Design review of the part built by this model. Coordinates are the model's own, in mm. A direction names the side the tool comes from. Give positions to 0.01 mm unless a question says otherwise; leave off trailing zeros. Order: outer loops, then holes, each group sorted by start corner. A loop starts at its lowest first (then second) coordinate and runs counter-clockwise, first axis right, second up. Notation, with made-up numbers: (-2, -35.75) -> (43, -35.75) arc R27 ccw to (43, 3.25) -> close; hole circle Ø4 at (71.5, -10). An arc over 180 degrees is marked (long way). One line per item, written item: value. Start each with the question number.
1) Consider section D-D (x = 3.5). State the section outline as (y, z) points, plus the area to 3 significant figures.
2) Consider section A-A (y = 0.9). State the section outline as (x, z) points, plus the area to 3 significant figures.
3) Consider section B-B (x = -15.25). State the section outline as (y, z) points, plus the area to 3 significant figures.
4) For pin 1 (11 mm diameter, centred on x = 3.5, z = -4, fed in from +Y); pin 2 (1 mm diameter, centred on y = 3, z = 3, fed in from -X); pin 3 (0.5 mm diameter, centred on x = 6.5, y = 2.5, fed in from +Z); pin 4 (1.1 mm diameter, centred on y = 2.5, z = 15.5, fed in from -X), all flat-tipped, find the tip position at first contact; note any pin that passes through.
5) The part is to be moulded in two halves that separate along Z. For faces 1 (the face through (0, 0, 0)), 2 (the face through (15.32, 0.86, -16.75)), 3 (the face through (-15.18, 0.86, -16.75)), 4 (the face through (17.43, 0.86, 17.4)), say which applies: released by +Z, released by -Z, zero draft, split by the parting line, or undercut.
6) Consider section C-C (z = -5.5). State the section outline as (x, y) points, plus the area to 3 significant figures.
7) Tool access review of faces 5 (the face through (7, 3, 15)), 6 (the face through (0, 1, -18)): name each direction out of +Z, -Z, +X, -X, +Y, -Y from which nothing blocks a thin tool from reaching the whole face with its end or side.
8) Wall thickness on line 1 along X through (y, z) = (1.45, 15.25); line 2 along Y through (x, z) = (0.5, -12): over which ranges is each line inside the solid? List them lowest first. Write a range as from..to.
from build123d import *

# Parameters (mm, degrees)
SKETCH2_R           = 1.5
BOSS_EXTRUDE1_DEPTH = 1.75
BOSS_EXTRUDE2_DEPTH = 3
BOSS_EXTRUDE3_DEPTH = 0.5
SKETCH6_R           = 0.25
CUT_EXTRUDE1_DEPTH  = 38.316216314


with BuildPart() as part:
    # Sketch2 → Boss-Extrude1 (new body)
    with BuildSketch(Plane(origin=(0, 0, 0), x_dir=(1, 0, 0), z_dir=(0, 1, 0))):
        with BuildLine():
            Line((16, -18), (-16, -18))
            ThreePointArc((-16, -18), (-17.414213562, -17.414213562), (-18, -16))
            Line((-18, -16), (-18, 16))
            ThreePointArc((-18, 16), (-17.414213562, 17.414213562), (-16, 18))
            Line((-16, 18), (16, 18))
            ThreePointArc((16, 18), (17.414213562, 17.414213562), (18, 16))
            Line((18, 16), (18, -16))
            ThreePointArc((18, -16), (17.414213562, -17.414213562), (16, -18))
        make_face()
        with Locations(Location((-15.25, 15.25, 0), (0, 0, 270))):
            Circle(SKETCH2_R, mode=Mode.SUBTRACT)
        with Locations(Location((15.25, 15.25, 0), (0, 0, 270))):
            Circle(SKETCH2_R, mode=Mode.SUBTRACT)
        with Locations(Location((15.25, -15.25, 0), (0, 0, 270))):
            Circle(SKETCH2_R, mode=Mode.SUBTRACT)
        with Locations(Location((-15.25, -15.25, 0), (0, 0, 270))):
            Circle(SKETCH2_R, mode=Mode.SUBTRACT)
    extrude(amount=BOSS_EXTRUDE1_DEPTH)

    # Sketch3 → Boss-Extrude2 (add)
    with BuildSketch(Plane.XY.offset(18)):
        with BuildLine():
            Line((5.557062961, 3.5), (8.150682516, 3.5))
            ThreePointArc((8.150682516, 3.5), (8.292103872, 3.441421356), (8.350682516, 3.3))
            Line((8.350682516, 3.3), (8.350682516, 3.184070744))
            ThreePointArc((8.350682516, 3.184070744), (8.40926116, 3.042649388), (8.550682516, 2.984070744))
            Line((8.550682516, 2.984070744), (8.650583865, 2.984070744))
            ThreePointArc((8.650583865, 2.984070744), (8.792005221, 2.925492101), (8.850583865, 2.784070744))
            Line((8.850583865, 2.784070744), (8.850583865, 1.75))
            Line((8.850583865, 1.75), (4.850583865, 1.75))
            Line((4.850583865, 1.75), (4.850583865, 2.784070744))
            ThreePointArc((4.850583865, 2.784070744), (4.909162509, 2.925492101), (5.050583865, 2.984070744))
            Line((5.050583865, 2.984070744), (5.157062961, 2.984070744))
            ThreePointArc((5.157062961, 2.984070744), (5.298484317, 3.042649388), (5.357062961, 3.184070744))
            Line((5.357062961, 3.184070744), (5.357062961, 3.3))
            ThreePointArc((5.357062961, 3.3), (5.415641605, 3.441421356), (5.557062961, 3.5))
        make_face()
        with BuildLine():
            Line((5.557062961, 3.4), (8.150682516, 3.4))
            ThreePointArc((8.150682516, 3.4), (8.221393194, 3.370710678), (8.250682516, 3.3))
            Line((8.250682516, 3.3), (8.250682516, 3.184070744))
            ThreePointArc((8.250682516, 3.184070744), (8.338550482, 2.97193871), (8.550682516, 2.884070744))
            Line((8.550682516, 2.884070744), (8.650583865, 2.884070744))
            ThreePointArc((8.650583865, 2.884070744), (8.721294543, 2.854781422), (8.750583865, 2.784070744))
            Line((8.750583865, 2.784070744), (8.750583865, 1.85))
            Line((8.750583865, 1.85), (4.950583865, 1.85))
            Line((4.950583865, 1.85), (4.950583865, 2.784070744))
            ThreePointArc((4.950583865, 2.784070744), (4.979873187, 2.854781422), (5.050583865, 2.884070744))
            Line((5.050583865, 2.884070744), (5.157062961, 2.884070744))
            ThreePointArc((5.157062961, 2.884070744), (5.369194995, 2.97193871), (5.457062961, 3.184070744))
            Line((5.457062961, 3.184070744), (5.457062961, 3.3))
            ThreePointArc((5.457062961, 3.3), (5.486352283, 3.370710678), (5.557062961, 3.4))
        make_face(mode=Mode.SUBTRACT)
    extrude(amount=-BOSS_EXTRUDE2_DEPTH)

    # Sketch5 → Boss-Extrude3 (add)
    with BuildSketch(Plane(origin=(0, 0, 15), x_dir=(-1, 0, 0), z_dir=(0, 0, -1))):
        with BuildLine():
            Line((-8.350682516, 3.3), (-8.350682516, 3.184070744))
            ThreePointArc((-8.350682516, 3.184070744), (-8.40926116, 3.042649388), (-8.550682516, 2.984070744))
            Line((-8.550682516, 2.984070744), (-8.650583865, 2.984070744))
            ThreePointArc((-8.650583865, 2.984070744), (-8.792005221, 2.925492101), (-8.850583865, 2.784070744))
            Line((-8.850583865, 2.784070744), (-8.850583865, 1.75))
            Line((-8.850583865, 1.75), (-4.850583865, 1.75))
            Line((-4.850583865, 1.75), (-4.850583865, 2.784070744))
            ThreePointArc((-4.850583865, 2.784070744), (-4.909162509, 2.925492101), (-5.050583865, 2.984070744))
            Line((-5.050583865, 2.984070744), (-5.157062961, 2.984070744))
            ThreePointArc((-5.157062961, 2.984070744), (-5.298484317, 3.042649388), (-5.357062961, 3.184070744))
            Line((-5.357062961, 3.184070744), (-5.357062961, 3.3))
            ThreePointArc((-5.357062961, 3.3), (-5.415641605, 3.441421356), (-5.557062961, 3.5))
            Line((-5.557062961, 3.5), (-8.150682516, 3.5))
            ThreePointArc((-8.150682516, 3.5), (-8.292103872, 3.441421356), (-8.350682516, 3.3))
        make_face()
    extrude(amount=BOSS_EXTRUDE3_DEPTH)

    # Sketch6 → Cut-Extrude1 (cut, through all)
    with BuildSketch(Plane(origin=(0, 0, 14.5), x_dir=(-1, 0, 0), z_dir=(0, 0, -1))):
        with Locations((-7.650583865, 2.218305959)):
            Circle(SKETCH6_R)
        with Locations((-6.850583865, 2.218305959)):
            Circle(SKETCH6_R)
        with Locations((-6.050583865, 2.218305959)):
            Circle(SKETCH6_R)
    extrude(amount=-CUT_EXTRUDE1_DEPTH, mode=Mode.SUBTRACT)


solid = part.part
Checked values:
1. outline: (0, -18) -> (1.75, -18) -> (1.75, 18) -> (0, 18) -> close
1. area: 63.0 mm^2
2. outline: (-18, -16) arc R2 ccw to (-16, -18) -> (16, -18) arc R2 ccw to (18, -16) -> (18, 16) arc R2 ccw to (16, 18) -> (-16, 18) arc R2 ccw to (-18, 16) -> close; hole circle Ø3 at (-15.25, -15.25); hole circle Ø3 at (-15.25, 15.25); hole circle Ø3 at (15.25, -15.25); hole circle Ø3 at (15.25, 15.25)
2. area: 1,260 mm^2
3. outline: (0, -18) -> (1.75, -18) -> (1.75, -16.75) -> (0, -16.75) -> close; (0, -13.75) -> (1.75, -13.75) -> (1.75, 13.75) -> (0, 13.75) -> close; (0, 16.75) -> (1.75, 16.75) -> (1.75, 18) -> (0, 18) -> close
3. area: 52.5 mm^2
4. pin 1: stops at y = 1.75
4. pin 2: passes through
4. pin 3: stops at z = 15
4. pin 4: stops at x = 4.85
5. face 1: zero draft
5. face 2: undercut
5. face 3: undercut
5. face 4: released by +Z
6. outline: (-18, 0) -> (18, 0) -> (18, 1.75) -> (-18, 1.75) -> close
6. area: 63.0 mm^2
7. face 5: +Z
7. face 6: -Z, +X, -X, +Y, -Y
8. line 1: x = -18..-16.75, -13.75..13.75, 16.75..18
8. line 2: y = 0..1.75
